Read the model definition and answer for the solid it produces. Units are mm, in the model's axes. Coordinates: 2 decimals unless noted, no trailing zeros. Write each loop counter-clockwise with the first axis right and the second up, starting at its lowest first coordinate (ties: lowest second). Pieces come first, ordered by that corner, then holes. Notation, with made-up numbers: (61, 3.5) -> (111, 3.5) arc R20 cw to (111, 30.5) -> close; hole circle Ø7 at (59, -27). An arc over 180 degrees is marked (long way). Answer in a Markdown table with one row per item. Add a question column.
Item 1: Given pin 1 Ø1 at (x, z) = (1.5, -13) entering from -Y, flat-ended and moving along its own axis, determine where the tip first touches the part or whether it passes through.
Item 2: Section A-A on z = -50 is taken. Write down the section's boundary in (x, y) (3 decimals).
Item 3: Section C-C on x = 2 is taken. Count the separate pieces of the cut face and the enclosed holes in it, then the cut area to 3 significant figures.
Item 4: Straight lines are drawn through the part: line 1 (Z direction, x = 2.05, y = 90) (3 decimals); line 2 (Y direction, x = 2.1, z = -12.5) (3 decimals); line 3 (Y direction, x = 1.3, z = -50). For each, find the intervals that lie inside material, in ascending order. Write a range as from..to.
Item 5: Section B-B on y = 15.5 is taken. Write down the section's boundary in (x, z) (3 decimals), then the cut area to 3 significant figures.
```python
from build123d import *

# Parameters (mm, degrees)
SKETCH1_W           = 100
SKETCH1_H           = 106.35
SKETCH1_R           = 5
SKETCH1_W_2         = 3.175
SKETCH1_H_2         = 10
SKETCH1_W_3         = 10
SKETCH1_H_3         = 3.175
BOSS_EXTRUDE1_DEPTH = 3.175


with BuildPart() as part:
    # Sketch1 → Boss-Extrude1 (new body)
    with BuildSketch(Plane(origin=(0, 0, 0), x_dir=(0, 0, -1), z_dir=(1, 0, 0))):
        with Locations((50, 53.175)):
            Rectangle(SKETCH1_W, SKETCH1_H)
        with Locations((50, 26.509283713)):
            Circle(SKETCH1_R, mode=Mode.SUBTRACT)
        with Locations((4.7625, 88.175)):
            Rectangle(SKETCH1_W_2, SKETCH1_H_2, mode=Mode.SUBTRACT)
        with Locations((15, 101.5875)):
            Rectangle(SKETCH1_W_3, SKETCH1_H_3, mode=Mode.SUBTRACT)
        with Locations((85, 101.5875)):
            Rectangle(SKETCH1_W_3, SKETCH1_H_3, mode=Mode.SUBTRACT)
        with Locations((95.2375, 88.175)):
            Rectangle(SKETCH1_W_2, SKETCH1_H_2, mode=Mode.SUBTRACT)
        with Locations((95.2375, 18.175)):
            Rectangle(SKETCH1_W_2, SKETCH1_H_2, mode=Mode.SUBTRACT)
        with Locations((85, 4.7625)):
            Rectangle(SKETCH1_W_3, SKETCH1_H_3, mode=Mode.SUBTRACT)
        with Locations((15, 4.7625)):
            Rectangle(SKETCH1_W_3, SKETCH1_H_3, mode=Mode.SUBTRACT)
        with Locations((4.7625, 18.175)):
            Rectangle(SKETCH1_W_2, SKETCH1_H_2, mode=Mode.SUBTRACT)
    extrude(amount=BOSS_EXTRUDE1_DEPTH)


solid = part.part
```
Results below:
| question | item | result |
|---|---|---|
| 1 | pin 1 | stops at y = 0 |
| 2 | outline | (0, 0) -> (3.175, 0) -> (3.175, 21.509) -> (0, 21.509) -> close; (0, 31.509) -> (3.175, 31.509) -> (3.175, 106.35) -> (0, 106.35) -> close |
| 3 | separate pieces | 1 |
| 3 | enclosed holes | 9 |
| 3 | area | 10,300 mm2 |
| 4 | line 1 | z = -100..-96.825, -93.65..-6.35, -3.175..0 |
| 4 | line 2 | y = 0..3.175, 6.35..100, 103.175..106.35 |
| 4 | line 3 | y = 0..21.51, 31.51..106.35 |
| 5 | outline | (0, -100) -> (3.175, -100) -> (3.175, -96.825) -> (0, -96.825) -> close; (0, -93.65) -> (3.175, -93.65) -> (3.175, -6.35) -> (0, -6.35) -> close; (0, -3.175) -> (3.175, -3.175) -> (3.175, 0) -> (0, 0) -> close |
| 5 | area | 297 mm2 |
